Input: part model. Units: mm. Frame: model coordinates. Give positions to 0.01 mm unless a question says otherwise; leave off trailing zeros. Loops run counter-clockwise (first coordinate to the right, second up) from the corner with the lowest first, then second, coordinate; pieces in that order, holes last. Notation, with made-up numbers: (18, -8.5) - (39, -8.5) arc R19 ccw to (39, 14.5) - close; hole circle Ø6 at (24.25, 52.5). An arc over 180 degrees is marked (long way). Answer as a JSON object with one key per item and string values.
from build123d import *

# Parameters (mm, degrees)
SKETCH1_W           = 120
SKETCH1_H           = 200
BOSS_EXTRUDE1_DEPTH = 40
BOSS_EXTRUDE2_DEPTH = 120
CUT_EXTRUDE2_DEPTH  = 1


with BuildPart() as part:
    # Sketch1 → Boss-Extrude1 (new body)
    with BuildSketch(Plane(origin=(0, 0, 0), x_dir=(1, 0, 0), z_dir=(0, 1, 0))):
        Rectangle(SKETCH1_W, SKETCH1_H)
    extrude(amount=BOSS_EXTRUDE1_DEPTH)

    # Sketch2 → Boss-Extrude2 (add)
    with BuildSketch(Plane(origin=(60, 0, 0), x_dir=(0, 0, -1), z_dir=(1, 0, 0))):
        Polygon((67.4, 40), (64.99822288, 44.16), (77.40177712, 44.16), (75, 40), align=None)
        Polygon((-75, 40), (-77.40177712, 44.16), (-64.99822288, 44.16), (-67.4, 40), align=None)
    extrude(amount=-BOSS_EXTRUDE2_DEPTH)

    # Sketch5 → Cut-Extrude2 (cut)
    with BuildSketch(Plane.XZ):
        Polygon((-10.888743303, -30.135074667), (-10.888743303, 13.324383252), (-25.483702069, 13.324383252), (0, 40.546241509), (25.483702069, 13.324383252), (10.888743303, 13.324383252), (10.888743303, -30.135074667), align=None)
    extrude(amount=-CUT_EXTRUDE2_DEPTH, mode=Mode.SUBTRACT)


solid = part.part
Item 1: Cut plane B-B (z = -83). Return loops of the section in (x, y).
Geometry check:
{"outline": "(-60, 0) - (60, 0) - (60, 40) - (-60, 40) - close"}
Item 2: Cut plane A-A (x = 29). Return loops of the section in (y, z).
Geometry check:
{"outline": "(0, -100) - (40, -100) - (40, -75) - (44.16, -77.4) - (44.16, -65) - (40, -67.4) - (40, 67.4) - (44.16, 65) - (44.16, 77.4) - (40, 75) - (40, 100) - (0, 100) - close"}
Item 3: Contact query for a flat-ended pin moving along its axis: P1, Ø5, axis at x = 26, z = 47, coming from the +Y side. Output: stop coordinate, or through.
Geometry check:
{"P1": "stops at y = 40"}
Item 4: Mould query, pull axis X, two halves, no side actions, for faces 1 (the face through (-60, 22, 1)), 2 (the face through (-12.92, 0.493, 26.745)), 3 (the face through (-1, 40, -1)), 4 (the face through (12.56, 0.49, 27.13)). Classes: released by +X, released by -X, zero draft, split by the parting line, or undercut.
Geometry check:
{"face 1": "released by -X", "face 2": "undercut", "face 3": "zero draft", "face 4": "undercut"}
Item 5: Material intervals for line 1 (Y direction, x = 31, z = -9.5); line 2 (Y direction, x = -4, z = 66.5), sorted ascending. Write a range as [from, to].
Geometry check:
{"line 1": "y = [0, 40]", "line 2": "y = [0, 40], [41.56, 44.16]"}
Item 6: Cut plane C-C (x = 14). Return loops of the section in (y, z).
Geometry check:
{"outline": "(0, -100) - (40, -100) - (40, -75) - (44.16, -77.4) - (44.16, -65) - (40, -67.4) - (40, 67.4) - (44.16, 65) - (44.16, 77.4) - (40, 75) - (40, 100) - (0, 100) - (0, 25.59) - (1, 25.59) - (1, 13.32) - (0, 13.32) - close"}
Item 7: Cut plane D-D (x = -2.5). Return loops of the section in (y, z).
Geometry check:
{"outline": "(0, -100) - (40, -100) - (40, -75) - (44.16, -77.4) - (44.16, -65) - (40, -67.4) - (40, 67.4) - (44.16, 65) - (44.16, 77.4) - (40, 75) - (40, 100) - (0, 100) - (0, 37.88) - (1, 37.88) - (1, -30.14) - (0, -30.14) - close"}
